Autodesk Inventor part; units mm, degrees
ref_plane "YZ Plane" through (0, 0, 0) normal (1, 0, 0) x (0, 1, 0)
ref_plane "XZ Plane" through (0, 0, 0) normal (0, 1, 0) x (-1, 0, 0)
ref_plane "XY Plane" through (0, 0, 0) normal (0, 0, 1) x (1, 0, 0)
sketch "Sketch1" plane through (0, 0, 0) normal (1, 0, 0) x (0, 1, 0)
  line L0 (3, 0) -> (15, 0)
  line L1 (15, 0) -> (15, -2.5)
  line L2 (15, -2.5) -> (13, -4)
  line L3 (13, -4) -> (12, -4)
  line L4 (12, -4) -> (12, -2.5)
  line L5 (0, -4) -> (0, 0)
  arc A0 (12, -2.5) -> (2.027, -4.1622) centre (12, -33.25) ccw
  line L6 (0, 3) -> (0, 0)
  arc A1 (0, 3) -> (3, 0) centre (3, 3) ccw
  line L7 (0, -4) -> (0, -7)
  arc A2 (2.027, -4.1622) -> (0, -7) centre (3, -7) ccw
  dimension "d0" = 12
  dimension "d1" = 4
  dimension "d2" = 1.5
  dimension "d3" = 3
  dimension "d4" = 2.5
  dimension "d5" = 1
  dimension "d15" = 3
  dimension "d17" = 3
  dimension "d18" = 3
extrude "Extrusion1" add sketch "Sketch1" along normal blind 5
properties part number "Clipje" material "ABS Plastic"
CAD build for the part. Positions are in the model's coordinates, mm. A direction names the side the tool comes from. Round coordinates to 2 decimals unless told otherwise and drop trailing zeros. Write each loop counter-clockwise with the first axis right and the second up, starting at its lowest first coordinate (ties: lowest second). Pieces come first, ordered by that corner, then holes. Notation, with made-up numbers: (64.25, 2.5) - (120.25, 2.5) arc R19 ccw to (120.25, 24.5) - close; hole circle Ø8 at (75.25, 25). An arc over 180 degrees is marked (long way). Write item = value, one per line. Start each with the question number.
Q1. Which spindle directions (+Z, -Z, +X, -X, +Y, -Y) get a long thin tool onto all of the face, cutting with end or side? Do faces 1 (the cylindrical face through (2.46, 6.87, -2.93)), 2 (the flat face through (2, 9, 0)), 3 (the flat face through (0, 6, -2)). Say none if no direction does.
Q2. Band-saw the part on D-D (z = -4.75). Give the cut face in (x, y).
Q3. Band-saw the part on B-B (x = 1.55). Give the cut face in (y, z).
Q4. Band-saw the part on A-A (z = -2.75). Give the cut face in (x, y), then the cut area to 3 significant figures.
Q5. Band-saw the part on C-C (y = 3.5). Give the cut face in (x, z).
Q6. Probe L1, parallel to Z at x = 1.95, y = 5; L2, parallel to Z at x = 4.7, y = 9.25; L3, parallel to Y at x = 2.05, z = 0.75. List the from-to ranges inside material, lowest first. Write a range as from..to.
Q7. Mould opens along Y. For faces 4 (the flat face through (2.5, 12.5, -4)), 5 (the flat face through (2.465, 14.014, -3.24)), 6 (the flat face through (2, 12, -3)) say: pulls with the +Y half, pulls with the -Y half, needs draft (parallel to the pull), parting line crosses it, or undercut.
Q8. Drop flat-ended pins along their axis: pin 1 (3 mm diameter, centred on x = 2.5, y = 4, fed in from +Z); pin 2 (0.8 mm diameter, centred on x = 2, y = 12.5, fed in from -Z). Give the stop position or say it passes through.
Answers below:
q1.face_1 = -Z, +X, -X
q1.face_2 = +Z, +X, -X, +Y
q1.face_3 = +Z, -Z, -X, +Y, -Y
q2.outline = (0, 0) - (5, 0) - (5, 1.02) - (0, 1.02) - close
q3.outline = (0, -7) arc R3 cw to (2.03, -4.16) arc R30.75 cw to (12, -2.5) - (12, -4) - (13, -4) - (15, -2.5) - (15, 0) - (3, 0) arc R3 cw to (0, 3) - close
q4.outline = (0, 0) - (5, 0) - (5, 8.09) - (0, 8.09) - close; (0, 12) - (5, 12) - (5, 14.67) - (0, 14.67) - close
q4.area = 53.8 mm2
q5.outline = (0, -3.7) - (5, -3.7) - (5, 0) - (0, 0) - close
q6.L1 = -3.31..0
q6.L2 = -2.62..0
q6.L3 = 0..1.02
q7.face_4 = needs draft
q7.face_5 = pulls with the +Y half
q7.face_6 = undercut
q8.pin_1 = 0.04
q8.pin_2 = -4
